Read the model definition and answer for the solid it produces. Units are mm, in the model's axes. A direction names the side the tool comes from. Give positions to 0.01 mm unless a question says otherwise; leave off trailing zeros. Loops run counter-clockwise (first coordinate to the right, second up) from the corner with the lowest first, then second, coordinate; pieces in that order, holes last. Notation, with made-up numbers: (49, 38) - (78, 38) arc R24 ccw to (78, 75) - close; hole circle Ø8 at (30, 23.5). An arc over 180 degrees is marked (long way). Write item = value, one per line.
```python
from build123d import *

# Parameters (mm, degrees)
SALIENTE_EXTRUIR1_DEPTH                              = 9.8
CORTAR_EXTRUIR1_DEPTH                                = 2.2
SALIENTE_EXTRUIR2_DEPTH                              = 2.2
SALIENTE_EXTRUIR3_DEPTH                              = 2.2
TALADRO_DE_MARGEN_PARA_M241_D                        = 27.8721
TALADRO_DE_MARGEN_PARA_M241_DEPTH                    = 0.3
CROQUIS7_W                                           = 10.5
CROQUIS7_H                                           = 2.86
REFRENTADO_PARA_PERNO_CON_CABEZA_HEXAGON_D           = 8.45
REFRENTADO_PARA_PERNO_CON_CABEZA_HEXAGON_CBORE_D     = 15
REFRENTADO_PARA_PERNO_CON_CABEZA_HEXAGON_CBORE_DEPTH = 8.8
DI_METRO_DE_TALADRO_3_0_3_1_D                        = 3
DI_METRO_DE_TALADRO_3_0_3_1_DEPTH                    = 10.16
CHAFL_N1_SIZE                                        = 0.25
REDONDEO1_R                                          = 1


with BuildPart() as part:
    # Croquis1 → Saliente-Extruir1 (new body)
    with BuildSketch(Plane(origin=(0, 0, 0), x_dir=(1, 0, 0), z_dir=(0, 1, 0))):
        Polygon((-21, 17), (-21, -17), (-17, -21), (17, -21), (21, -17), (21, 17), (17, 21), (-17, 21), align=None)
    extrude(amount=-SALIENTE_EXTRUIR1_DEPTH)

    # Croquis2 → Cortar-Extruir1 (cut)
    with BuildSketch(Plane(origin=(0, 0, 0), x_dir=(-1, 0, 0), z_dir=(0, 1, 0))):
        Polygon((-14.100780618, -21), (14.100780618, -21), (21, -14.100780618), (21, 17), (17, 21), (-17, 21), (-21, 17), (-21, -14.100780618), align=None)
    extrude(amount=-CORTAR_EXTRUIR1_DEPTH, mode=Mode.SUBTRACT)

    # Croquis3 → Saliente-Extruir2 (add)
    with BuildSketch(Plane(origin=(0, -2.2, 0), x_dir=(-1, 0, 0), z_dir=(0, 1, 0))):
        Polygon((-14.100780618, 21), (-21, 14.100780618), (-21, 17), (-17, 21), align=None)
    extrude(amount=SALIENTE_EXTRUIR2_DEPTH)

    # Croquis4 → Saliente-Extruir3 (add)
    with BuildSketch(Plane(origin=(0, -2.2, 0), x_dir=(-1, 0, 0), z_dir=(0, 1, 0))):
        Polygon((17, 21), (21, 17), (21, 14.100780618), (14.100780618, 21), align=None)
    extrude(amount=SALIENTE_EXTRUIR3_DEPTH)

    # Taladro de margen para M241
    with Locations(Plane(origin=(0, -9.8, 0), x_dir=(-1, 0, 0), z_dir=(0, -1, 0))):
        with Locations((0, 0)):
            Hole(TALADRO_DE_MARGEN_PARA_M241_D / 2, depth=TALADRO_DE_MARGEN_PARA_M241_DEPTH)

    # Croquis7 → Revolución1 (revolve)
    with BuildSketch(Plane.XY, mode=Mode.PRIVATE) as revoluci_n1_sk:
        with Locations((5.25, -10.93)):
            Rectangle(CROQUIS7_W, CROQUIS7_H)
    revolve(revoluci_n1_sk.sketch.rotate(Axis((0, -9.5, 0), (0, -1, 0)), 270), axis=Axis((0, -9.5, 0), (0, -1, 0)))

    # Refrentado para perno con cabeza hexagonal de M81 (through all)
    with Locations(Plane(origin=(0, -2.2, 0), x_dir=(1, 0, 0), z_dir=(0, 1, 0))):
        with Locations((0, 0)):
            CounterBoreHole(REFRENTADO_PARA_PERNO_CON_CABEZA_HEXAGON_D / 2, REFRENTADO_PARA_PERNO_CON_CABEZA_HEXAGON_CBORE_D / 2, REFRENTADO_PARA_PERNO_CON_CABEZA_HEXAGON_CBORE_DEPTH)

    # Diámetro de taladro Ø3.0 (3)1
    with Locations(Plane(origin=(0, -2.2, 0), x_dir=(1, 0, 0), z_dir=(0, 1, 0))):
        with Locations((15.5, -15.5), (15.5, 15.5), (-15.5, -15.5), (-15.5, 15.5)):
            Hole(DI_METRO_DE_TALADRO_3_0_3_1_D / 2, depth=DI_METRO_DE_TALADRO_3_0_3_1_DEPTH)

    # Chaflán1
    chafl_n1_edges = [part.edges().sort_by_distance(p)[0] for p in [
        (4.225, -12.36, 0),
    ]]
    chamfer(chafl_n1_edges, length=CHAFL_N1_SIZE)

    # Redondeo1
    redondeo1_edges = [part.edges().sort_by_distance(p)[0] for p in [
        (-17, -4.9, -21),
        (17, -4.9, -21),
        (21, -4.9, -17),
        (21, -4.9, 17),
        (17, -4.9, 21),
        (-17, -4.9, 21),
        (-21, -4.9, 17),
        (-21, -4.9, -17),
    ]]
    fillet(redondeo1_edges, radius=REDONDEO1_R)


solid = part.part
```
1) Find the intervals of material crossed by probe 1 along Z at (x, y) = (15.5, -7.25); probe 2 along X at (y, z) = (-11.25, 0) (3 decimals), in increasing order.
Output:
probe_1 = -21 to -17, -14 to 14, 17 to 21
probe_2 = -10.5 to -4.225, 4.225 to 10.5
2) The mould has two halves that part along X. Classify faces 4 (the face through (-14, -6.05, 15.43)), 5 (the face through (18, 0, -18)), 6 (the face through (19, -5, 19)), 7 (the face through (10, -2.2, 0)): pulls with the +X half, pulls with the -X half, needs draft (parallel to the pull), parting line crosses it, or undercut.
Output:
face_4 = undercut
face_5 = needs draft
face_6 = pulls with the +X half
face_7 = undercut
3) Each of these flat-tipped pins is pushed along its axis until it touches: P1, Ø9, axis at x = 0, z = 0, coming from the -Y side; P2, Ø1.8, axis at x = 15.5, z = 15.5, coming from the +Y side; P3, Ø4, axis at x = 8, z = -13, coming from the -Y side; P4, Ø4, axis at x = 1, z = -10, coming from the +Y side. Where does it stop, or does it pass through?
Output:
P1 = -12.36
P2 = through
P3 = -9.8
P4 = -2.2
4) A tool of negligible diameter and unlimited length cuts with its end or side. For faces 1 (the face through (17.5, -1.1, 17.6)), 2 (the face through (-11.06, -9.65, 8.48)), 3 (the face through (-18, 0, 18)), from which of +Z, -Z, +X, -X, +Y, -Y can it reach the whole face along a straight path? Write none if from no direction.
Output:
face_1 = +Y
face_2 = -Y
face_3 = +Z, -Z, +X, -X, +Y
5) A cutting plane is placed at C-C on z = 0. Determine the outline of the cut face in (x, y) (3 decimals).
Output:
outline = (-21, -9.8) - (-13.936, -9.8) - (-13.936, -9.5) - (-10.5, -9.5) - (-10.5, -12.36) - (-4.475, -12.36) - (-4.225, -12.11) - (-4.225, -11) - (-7.5, -11) - (-7.5, -2.2) - (-21, -2.2) - close; (4.225, -12.11) - (4.475, -12.36) - (10.5, -12.36) - (10.5, -9.5) - (13.936, -9.5) - (13.936, -9.8) - (21, -9.8) - (21, -2.2) - (7.5, -2.2) - (7.5, -11) - (4.225, -11) - close
6) A cutting plane is placed at B-B on y = -1.5. Determine the outline of the cut face in (x, z), then the cut area to 3 significant figures.
Output:
outline = (-21, -16.59) arc R1 ccw to (-20.71, -17.29) - (-17.29, -20.71) arc R1 ccw to (-16.59, -21) - (-14.1, -21) - (-21, -14.1) - close; (-21, 14.1) - (-14.1, 21) - (-16.59, 21) arc R1 ccw to (-17.29, 20.71) - (-20.71, 17.29) arc R1 ccw to (-21, 16.59) - close; (14.1, -21) - (16.59, -21) arc R1 ccw to (17.29, -20.71) - (20.71, -17.29) arc R1 ccw to (21, -16.59) - (21, -14.1) - close; (14.1, 21) - (21, 14.1) - (21, 16.59) arc R1 ccw to (20.71, 17.29) - (17.29, 20.71) arc R1 ccw to (16.59, 21) - close
area = 63.0 mm²
7) A cutting plane is placed at A-A on x = 0. Determine the outline of the cut face in (y, z) (3 decimals), then the cut area to 3 significant figures.
Output:
outline = (-12.36, -10.5) - (-9.5, -10.5) - (-9.5, -13.936) - (-9.8, -13.936) - (-9.8, -21) - (-2.2, -21) - (-2.2, -7.5) - (-11, -7.5) - (-11, -4.225) - (-12.11, -4.225) - (-12.36, -4.475) - close; (-12.36, 4.475) - (-12.11, 4.225) - (-11, 4.225) - (-11, 7.5) - (-2.2, 7.5) - (-2.2, 21) - (-9.8, 21) - (-9.8, 13.936) - (-9.5, 13.936) - (-9.5, 10.5) - (-12.36, 10.5) - close
area = 227 mm²
8) A cutting plane is placed at D-D on x = -15.5. Determine the outline of the cut face in (y, z).
Output:
outline = (-9.8, -21) - (0, -21) - (0, -19.6) - (-2.2, -19.6) - (-2.2, -17) - (-9.8, -17) - close; (-9.8, -14) - (-2.2, -14) - (-2.2, 14) - (-9.8, 14) - close; (-9.8, 17) - (-2.2, 17) - (-2.2, 19.6) - (0, 19.6) - (0, 21) - (-9.8, 21) - close
